Source: CAD feature listing. Evaluate the final solid. Frame: model axes, mm. Face numbers are marked on the shaded views. A direction names the side the tool comes from. Coordinates: 2 decimals unless noted, no trailing zeros. Order: outer loops, then holes, each group sorted by start corner. A loop starts at its lowest first (then second) coordinate and runs counter-clockwise, first axis right, second up. Notation, with made-up numbers: (-32.75, 49.5) -> (11.25, 49.5) arc R23 ccw to (11.25, 80.5) -> close; hole circle Ø2 at (51, 35). An arc over 180 degrees is marked (long way). Put each result on its own line as item: value.
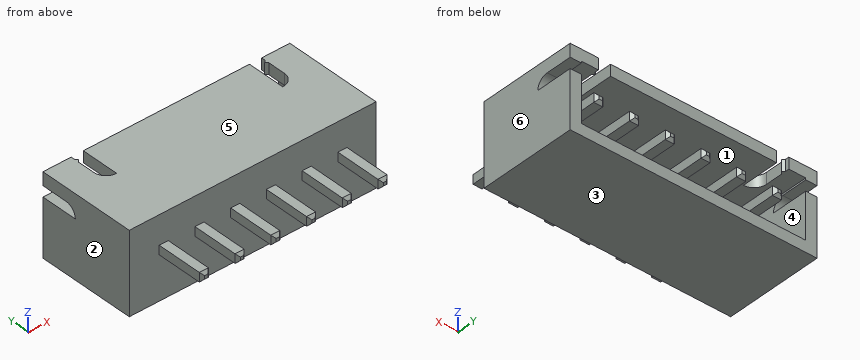
from build123d import *

# Parameters (mm, degrees)
SKETCH1_W                = 17.54
SKETCH1_H                = 5.75
BOSS_EXTRUDE1_DEPTH      = 7
SHELL1_T                 = -0.8
CUT_EXTRUDE1_DEPTH       = 18.54
CUT_EXTRUDE2_REACH       = 7.75
SKETCH4_W                = 0.64
SKETCH4_H                = 0.64
BOSS_EXTRUDE2_DEPTH      = 3.45
BOSS_EXTRUDE2_DEPTH_BACK = 6.75
CHAMFER1_SIZE            = 0.2


with BuildPart() as part:
    # Sketch1 → Boss-Extrude1 (new body)
    with BuildSketch(Plane(origin=(0, 0, 0), x_dir=(1, 0, 0), z_dir=(0, 1, 0))):
        Rectangle(SKETCH1_W, SKETCH1_H)
    extrude(amount=BOSS_EXTRUDE1_DEPTH)

    # Shell1
    shell1_openings = [part.faces().sort_by_distance(p)[0] for p in [
        (0, 7, 0),
    ]]
    offset(amount=SHELL1_T, openings=shell1_openings, kind=Kind.INTERSECTION)

    # Sketch2 → Cut-Extrude1 (cut, through all)
    with BuildSketch(Plane(origin=(8.77, 0, 0), x_dir=(0, 0, -1), z_dir=(1, 0, 0))):
        with BuildLine():
            Line((-1.19301282, 7), (-1.19301282, 4.379603984))
            ThreePointArc((-1.19301282, 4.379603984), (-1.72610374, 4.600417472), (-1.946917229, 5.133508392))
            Line((-1.946917229, 5.133508392), (-1.946917229, 7))
            Line((-1.946917229, 7), (-1.19301282, 7))
        make_face()
    extrude(amount=-CUT_EXTRUDE1_DEPTH, mode=Mode.SUBTRACT)

    # Sketch3 → Cut-Extrude2 (cut, up to next)
    with BuildSketch(Plane.XY.offset(2.875), mode=Mode.PRIVATE) as cut_extrude2_sk1:
        with BuildLine():
            Line((-6.77, 7), (-6.77, 6.728922615))
            Line((-6.77, 6.728922615), (-6.617135549, 6.576058164))
            Line((-6.617135549, 6.576058164), (-6.77, 6.423193713))
            Line((-6.77, 6.423193713), (-6.77, 5.166308225))
            ThreePointArc((-6.77, 5.166308225), (-6.516286554, 4.553789782), (-5.90376811, 4.300076336))
            Line((-5.90376811, 4.300076336), (-5.90376811, 7))
            Line((-5.90376811, 7), (-6.77, 7))
        make_face()
    cut_extrude2_tool1 = extrude(cut_extrude2_sk1.sketch, amount=-CUT_EXTRUDE2_REACH, mode=Mode.PRIVATE) & part.part
    add(cut_extrude2_tool1.solids().sort_by_distance((-6.314828, 5.726435, 2.875))[0], mode=Mode.SUBTRACT)
    # Sketch3 → Cut-Extrude2 (cut, up to next)
    with BuildSketch(Plane.XY.offset(2.875), mode=Mode.PRIVATE) as cut_extrude2_sk2:
        with BuildLine():
            Line((5.90376811, 7), (6.77, 7))
            Line((6.77, 7), (6.77, 6.728922615))
            Line((6.77, 6.728922615), (6.617135549, 6.576058164))
            Line((6.617135549, 6.576058164), (6.77, 6.423193713))
            Line((6.77, 6.423193713), (6.77, 5.166308225))
            ThreePointArc((6.77, 5.166308225), (6.516286554, 4.553789782), (5.90376811, 4.300076336))
            Line((5.90376811, 4.300076336), (5.90376811, 7))
        make_face()
    cut_extrude2_tool2 = extrude(cut_extrude2_sk2.sketch, amount=-CUT_EXTRUDE2_REACH, mode=Mode.PRIVATE) & part.part
    add(cut_extrude2_tool2.solids().sort_by_distance((6.314828, 5.726435, 2.875))[0], mode=Mode.SUBTRACT)

    # Sketch4 → Boss-Extrude2 (add, two sides)
    with BuildSketch(Plane.XZ) as boss_extrude2_sk:
        with Locations((-6.32, 0.525)):
            Rectangle(SKETCH4_W, SKETCH4_H)
        with Locations((-3.78, 0.525)):
            Rectangle(SKETCH4_W, SKETCH4_H)
        with Locations((-1.24, 0.525)):
            Rectangle(SKETCH4_W, SKETCH4_H)
        with Locations((1.3, 0.525)):
            Rectangle(SKETCH4_W, SKETCH4_H)
        with Locations((3.84, 0.525)):
            Rectangle(SKETCH4_W, SKETCH4_H)
        with Locations((6.38, 0.525)):
            Rectangle(SKETCH4_W, SKETCH4_H)
    extrude(amount=BOSS_EXTRUDE2_DEPTH)
    extrude(boss_extrude2_sk.sketch, amount=-BOSS_EXTRUDE2_DEPTH_BACK)

    # Chamfer1
    chamfer1_edges = [part.edges().sort_by_distance(p)[0] for p in [
        (-6, 6.75, 0.525),
        (-6.32, 6.75, 0.205),
        (-6.64, 6.75, 0.525),
        (-6.32, 6.75, 0.845),
        (-6, -3.45, 0.525),
        (-6.32, -3.45, 0.845),
        (-6.64, -3.45, 0.525),
        (-6.32, -3.45, 0.205),
        (-3.78, 6.75, 0.205),
        (-4.1, 6.75, 0.525),
        (-3.78, 6.75, 0.845),
        (-3.46, 6.75, 0.525),
        (-3.78, -3.45, 0.205),
        (-3.46, -3.45, 0.525),
        (-3.78, -3.45, 0.845),
        (-4.1, -3.45, 0.525),
        (-1.24, 6.75, 0.205),
        (-1.56, 6.75, 0.525),
        (-1.24, 6.75, 0.845),
        (-0.92, 6.75, 0.525),
        (-1.24, -3.45, 0.205),
        (-0.92, -3.45, 0.525),
        (-1.24, -3.45, 0.845),
        (-1.56, -3.45, 0.525),
        (1.3, 6.75, 0.205),
        (0.98, 6.75, 0.525),
        (1.3, 6.75, 0.845),
        (1.62, 6.75, 0.525),
        (1.3, -3.45, 0.205),
        (1.62, -3.45, 0.525),
        (1.3, -3.45, 0.845),
        (0.98, -3.45, 0.525),
        (3.84, 6.75, 0.205),
        (3.52, 6.75, 0.525),
        (3.84, 6.75, 0.845),
        (4.16, 6.75, 0.525),
        (3.84, -3.45, 0.205),
        (4.16, -3.45, 0.525),
        (3.84, -3.45, 0.845),
        (3.52, -3.45, 0.525),
        (6.38, 6.75, 0.205),
        (6.06, 6.75, 0.525),
        (6.38, 6.75, 0.845),
        (6.7, 6.75, 0.525),
        (6.38, -3.45, 0.205),
        (6.7, -3.45, 0.525),
        (6.38, -3.45, 0.845),
        (6.06, -3.45, 0.525),
    ]]
    chamfer(chamfer1_edges, length=CHAMFER1_SIZE)


solid = part.part
1. First-contact query: pin 1 (0.5 mm diameter, centred on x = 6.5, y = -2.5, fed in from -Z) (3 decimals); pin 2 (1.5 mm diameter, centred on x = 6.5, z = -0.5, fed in from -Y) (3 decimals); pin 3 (0.7 mm diameter, centred on y = -2, z = 0.5, fed in from -X). Flat tips, straight axial feed; report the tip coordinate or a pass-through.
Numbers:
pin 1: stops at z = 0.205
pin 2: stops at y = -3.295
pin 3: stops at x = -6.64
2. Ray query, line 1 along Z through (x, y) = (-6.25, 3.5) (3 decimals); line 2 along X through (y, z) = (1, 1.4); line 3 along Z through (x, y) = (-4.25, 2.5) (3 decimals). Return the intervals inside material, ascending.
Numbers:
line 1: z = -2.875 to -2.075, 0.205 to 0.845, 2.075 to 2.875
line 2: x = -8.77 to -7.97, 7.97 to 8.77
line 3: z = -2.875 to -2.075, 2.075 to 2.875
3. Set-up query: the marked faces 1 and 2. Return all of +Z, -Z, +X, -X, +Y, -Y with unobstructed straight access to the full face (end or side cutting, diameter ignored); none if empty.
Numbers:
face 1: +Y
face 2: +Z, -Z, -X, +Y, -Y
4. Cut plane A-A on y = 4. Count the separate pieces of the cut face and the enclosed holes in it, plus the area to 3 significant figures.
Numbers:
separate pieces: 7
enclosed holes: 1
area: 37.2 mm2
5. Pull-direction query (Z, two-part tool) for the marked faces 3, 4, 5 and 6; classes: pulls with the +Z half, pulls with the -Z half, needs draft (parallel to the pull), parting line crosses it, or undercut.
Numbers:
face 3: pulls with the -Z half
face 4: undercut
face 5: pulls with the +Z half
face 6: needs draft
6. Cut plane C-C on z = -1. Output: boundary loops of the cut face in (x, y), plus the area to 3 significant figures.
Numbers:
outline: (-8.77, 0) -> (8.77, 0) -> (8.77, 7) -> (7.97, 7) -> (7.97, 0.8) -> (-7.97, 0.8) -> (-7.97, 7) -> (-8.77, 7) -> close
area: 24.0 mm2
7. Cut plane B-B on y = -2.5. Output: boundary loops of the cut face in (x, z) (3 decimals), plus the area to 3 significant figures.
Numbers:
outline: (-6.64, 0.205) -> (-6, 0.205) -> (-6, 0.845) -> (-6.64, 0.845) -> close; (-4.1, 0.205) -> (-3.46, 0.205) -> (-3.46, 0.845) -> (-4.1, 0.845) -> close; (-1.56, 0.205) -> (-0.92, 0.205) -> (-0.92, 0.845) -> (-1.56, 0.845) -> close; (0.98, 0.205) -> (1.62, 0.205) -> (1.62, 0.845) -> (0.98, 0.845) -> close; (3.52, 0.205) -> (4.16, 0.205) -> (4.16, 0.845) -> (3.52, 0.845) -> close; (6.06, 0.205) -> (6.7, 0.205) -> (6.7, 0.845) -> (6.06, 0.845) -> close
area: 2.46 mm2
8. Cut plane D-D on x = -5. Output: boundary loops of the cut face in (y, z) (3 decimals).
Numbers:
outline: (0, -2.875) -> (7, -2.875) -> (7, -2.075) -> (0.8, -2.075) -> (0.8, 2.075) -> (7, 2.075) -> (7, 2.875) -> (0, 2.875) -> close
